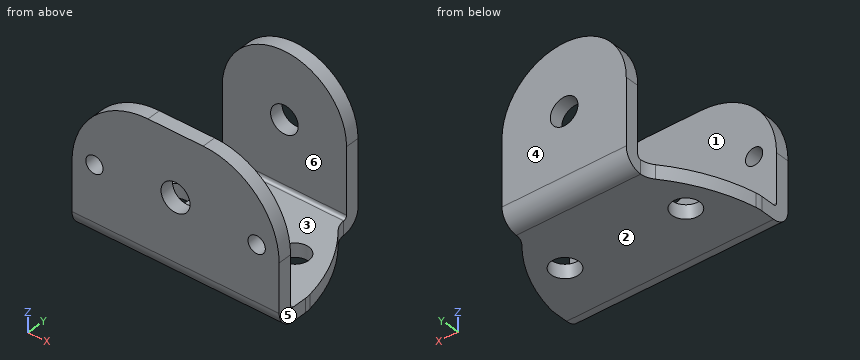
from build123d import *

# Parameters (mm, degrees)
BRIDA_BASE1_DEPTH                = 2
REDONDEO5MM_R                    = 5
REDONDEO3MM_R                    = 3
BRIDA_DE_ARISTA1_STRIP_W         = 9
BRIDA_DE_ARISTA1_STRIP_H         = 2
BRIDA_DE_ARISTA1_STRIP_CUT_DEPTH = 30
BRIDA_DE_ARISTA1_DEPTH           = 30
BRIDA_DE_ARISTA2_DEPTH           = 18
BRIDA_START                      = 2
BRIDA_DE_ARISTA2_FLAT_DEPTH      = 2
CORTAR_EXTRUIR6_REACH            = 43.255
CROQUIS26_R                      = 2
REDONDEO11MM_R                   = 11
TALADRO_ROSCADO_M32_D            = 2.5
TALADRO_ROSCADO_M32_DEPTH        = 20.65
TALADRO_ROSCADO_M32_TIP          = 0.751075774
TALADRO_ROSCADO_M52_D            = 4.2
TALADRO_ROSCADO_M52_DEPTH        = 2
CORTAR_EXTRUIR7_REACH            = 42.274
CROQUIS36_R                      = 2


# Sheet-metal steps are written as plain solids
with BuildPart() as part:
    # Croquis1 → Brida base1 (new body)
    with BuildSketch(Plane.XY):
        with BuildLine():
            Line((0, 0), (30, 0))
            Line((30, 0), (30, 3))
            ThreePointArc((30, 3), (27.901523057, 9.682731068), (24, 15.5))
            Line((24, 15.5), (24, 16.5))
            Line((24, 16.5), (6, 16.5))
            Line((6, 16.5), (6, 15.5))
            ThreePointArc((6, 15.5), (2.098476943, 9.682731068), (0, 3))
            Line((0, 3), (0, 0))
        make_face()
    extrude(amount=-BRIDA_BASE1_DEPTH)

    # Redondeo5mm
    redondeo5mm_edges = [part.edges().sort_by_distance(p)[0] for p in [
        (0, 3, -1),
        (30, 3, -1),
    ]]
    fillet(redondeo5mm_edges, radius=REDONDEO5MM_R)

    # Redondeo3mm
    # the kernel refuses this fillet: 3 mm, written as the material it adds along each edge
    with BuildSketch(Plane(origin=(24, 15.5, 0), x_dir=(0, 1, 0), z_dir=(0, 0, -1))) as redondeo3mm_piece_1:
        with BuildLine():
            CenterArc((1.118262022, 2.997668109), REDONDEO3MM_R, 230.394906527, 37.345869832)
            Line((-0.794215431, 0.686298387), (-0.83246498, 0.640070993))
            ThreePointArc((-0.83246498, 0.640070993), (-0.432666371, 0.301999114), (-0.040192089, -0.044548805))
            Line((-0.040192089, -0.044548805), (0, -0.06))
            ThreePointArc((0, -0.06), (0.5, -0.06), (0.99763476, -0.059953362))
            Line((0.99763476, -0.059953362), (1, 0))
        make_face()
    extrude(amount=2)
    with BuildSketch(Plane(origin=(6, 15.5, 0), x_dir=(-0.6538299662985165, -0.75664151034032, 0), z_dir=(0, 0, -1))) as redondeo3mm_piece_2:
        with BuildLine():
            CenterArc((1.113841774, 2.999313346), REDONDEO3MM_R, 231.428232408, 37.345869832)
            Line((-0.75664151, 0.653829966), (-0.794051176, 0.606920299))
            ThreePointArc((-0.794051176, 0.606920299), (-0.417550553, 0.281516493), (-0.039229798, -0.045398491))
            Line((-0.039229798, -0.045398491), (0.001283659, -0.059986267))
            ThreePointArc((0.001283659, -0.059986267), (0.524829407, -0.054385173), (1.048375155, -0.059986267))
            Line((1.048375155, -0.059986267), (1.049658814, 0))
        make_face()
    extrude(amount=2)

    # Brida de arista1 strip (across the edge) → Brida de arista1 strip cut (cut)
    with BuildSketch(Plane.YZ):
        with Locations((-4, -1)):
            Rectangle(BRIDA_DE_ARISTA1_STRIP_W, BRIDA_DE_ARISTA1_STRIP_H)
    extrude(amount=BRIDA_DE_ARISTA1_STRIP_CUT_DEPTH, mode=Mode.SUBTRACT)

    # Brida de arista1 section (across the edge) → Brida de arista1 (add)
    with BuildSketch(Plane.YZ):
        with BuildLine():
            Line((-2, 0.5), (-2, 18.5))
            Line((-2, 18.5), (0, 18.5))
            Line((0, 18.5), (0, 0.5))
            ThreePointArc((0, 0.5), (0.146446609, 0.146446609), (0.5, 0))
            Line((0.5, 0), (0.5, -2))
            ThreePointArc((0.5, -2), (-1.267766953, -1.267766953), (-2, 0.5))
        make_face()
    extrude(amount=BRIDA_DE_ARISTA1_DEPTH)

    # Brida de arista2 bend section (across the edge) → Brida de arista2 (add)
    with BuildSketch(Plane(origin=(24, 17, 0), x_dir=(0, -1, 0), z_dir=(-1, 0, 0))):
        with BuildLine():
            Line((-2, 0.5), (0, 0.5))
            ThreePointArc((0, 0.5), (0.146446609, 0.146446609), (0.5, 0))
            Line((0.5, 0), (0.5, -2))
            ThreePointArc((0.5, -2), (-1.267766953, -1.267766953), (-2, 0.5))
        make_face()
    extrude(amount=BRIDA_DE_ARISTA2_DEPTH)

    # Brida de arista2 profile (on flange) → Brida de arista2 flat (add)
    with BuildSketch(Plane(origin=(0, 17, 0), x_dir=(-1, 0, 0), z_dir=(0, 1, 0)).offset(BRIDA_START)):
        with BuildLine():
            ThreePointArc((-6, 10), (-15, 19), (-24, 10))
            Line((-24, 10), (-24, 0.5))
            Line((-24, 0.5), (-6, 0.5))
            Line((-6, 0.5), (-6, 10))
        make_face()
    extrude(amount=-BRIDA_DE_ARISTA2_FLAT_DEPTH)

    # Croquis26 → Cortar-Extruir6 (cut, up to next)
    with BuildSketch(Plane(origin=(0, 0, -2), x_dir=(-1, 0, 0), z_dir=(0, 0, -1)), mode=Mode.PRIVATE) as cortar_extruir6_sk1:
        with Locations((-6.25, 8.3)):
            Circle(CROQUIS26_R)
    cortar_extruir6_tool1 = extrude(cortar_extruir6_sk1.sketch, amount=-CORTAR_EXTRUIR6_REACH, mode=Mode.PRIVATE) & part.part
    # Croquis26 → Cortar-Extruir6 (cut, up to next)
    with BuildSketch(Plane(origin=(0, 0, -2), x_dir=(-1, 0, 0), z_dir=(0, 0, -1)), mode=Mode.PRIVATE) as cortar_extruir6_sk2:
        with Locations((-23.75, 8.3)):
            Circle(CROQUIS26_R)
    cortar_extruir6_tool2 = extrude(cortar_extruir6_sk2.sketch, amount=-CORTAR_EXTRUIR6_REACH, mode=Mode.PRIVATE) & part.part
    add(cortar_extruir6_tool1.solids().sort_by_distance((6.25, 8.3, -2))[0], mode=Mode.SUBTRACT)
    add(cortar_extruir6_tool2.solids().sort_by_distance((23.75, 8.3, -2))[0], mode=Mode.SUBTRACT)

    # Redondeo11mm
    redondeo11mm_edges = [part.edges().sort_by_distance(p)[0] for p in [
        (0, -1, 18.5),
        (30, -1, 18.5),
    ]]
    fillet(redondeo11mm_edges, radius=REDONDEO11MM_R)

    # Taladro roscado M32
    with Locations(Plane(origin=(0, 0, 0), x_dir=(1, 0, 0), z_dir=(0, 1, 0))):
        with Locations((3.25, -8.5), (26.75, -8.5)):
            Hole(TALADRO_ROSCADO_M32_D / 2, depth=TALADRO_ROSCADO_M32_DEPTH)
            with Locations((0, 0, -(TALADRO_ROSCADO_M32_DEPTH + TALADRO_ROSCADO_M32_TIP / 2))):  # 118° drill point
                Cone(0, TALADRO_ROSCADO_M32_D / 2, TALADRO_ROSCADO_M32_TIP, mode=Mode.SUBTRACT)

    # Taladro roscado M52
    with Locations(Plane(origin=(3.715500562, 0, 2.638137214), x_dir=(1, 0, 0), z_dir=(0, 1, 0))):
        with Locations((11.284499438, -6.861862786)):
            Hole(TALADRO_ROSCADO_M52_D / 2, depth=TALADRO_ROSCADO_M52_DEPTH)

    # Croquis36 → Cortar-Extruir7 (cut, up to next)
    with BuildSketch(Plane(origin=(0, 17, 0), x_dir=(1, 0, 0), z_dir=(0, 1, 0)), mode=Mode.PRIVATE) as cortar_extruir7_sk1:
        with Locations(Location((15, -9.5, 0), (0, 0, 270))):
            Circle(CROQUIS36_R)
    cortar_extruir7_tool1 = extrude(cortar_extruir7_sk1.sketch, amount=CORTAR_EXTRUIR7_REACH, mode=Mode.PRIVATE) & part.part
    add(cortar_extruir7_tool1.solids().sort_by_distance((15, 17, 9.5))[0], mode=Mode.SUBTRACT)


solid = part.part
Work out the finished part from the listing and answer in its coordinate system (mm). Face numbers are marked on the shaded views. A direction names the side the tool comes from. Coordinates: 2 decimals unless noted, no trailing zeros. Write each loop counter-clockwise with the first axis right and the second up, starting at its lowest first coordinate (ties: lowest second). Pieces come first, ordered by that corner, then holes. Notation, with made-up numbers: M -9.5,14 L 6.5,14 A7 cw 6.5,22 Z; hole C -12.5,-3.5 d10. An arc over 180 degrees is marked long. Answer as CSV lines item,"result". Start each with the question number.
Item 1: Section A-A on x = 15 is taken. Write down the section's boundary in (y, z), and give its area (3 significant figures).
Item 2: Consider L1, parallel to Y at x = 14.25, z = 1; L2, parallel to X at y = 18.15, z = 9.5; L3, parallel to X at y = -1, z = 8.5. Determine where each line is inside the solid, lowest interval first.
Item 3: Section C-C on y = 7 is taken. Write down the section's boundary in (x, z).
Item 4: Section B-B on x = 23 is taken. Write down the section's boundary in (y, z).
Item 5: Section D-D on z = 8.5 is taken. Write down the section's boundary in (x, y).
Item 6: Flat-ended cylindrical pins translate along their axes: P1, Ø4, axis at y = 8, z = 1, coming from the -X side; P2, Ø1, axis at x = 16.5, y = 10.5, coming from the +Z side; P3, Ø0.8, axis at y = 17.5, z = 3.5, coming from the +X side; P4, Ø2, axis at x = 3.25, z = 8.5, coming from the +Y side. Find the tip coordinate at first contact, or state that the pin passes through.
Item 7: A tool of negligible diameter and unlimited length cuts with its end or side. For the marked faces 5 and 6, from which of +Z, -Z, +X, -X, +Y, -Y can it reach the whole face along a straight path? Write none if from no direction.
Item 8: Determine the mould class of the marked faces 1, 2, 3 and 4 for opening direction Y: released by +Y, released by -Y, zero draft, split by the parting line, or undercut.
Checks:
1,outline,"M -2,0.5 A2.5 ccw 0.5,-2 L 16.5,-2 A2.5 ccw 19,0.5 L 19,7.5 L 17,7.5 L 17,0.5 A0.5 cw 16.5,0 L 0.5,0 A0.5 cw 0,0.5 L 0,7.4 L -2,7.4 Z; M -2,11.6 L 0,11.6 L 0,18.5 L -2,18.5 Z; M 17,11.5 L 19,11.5 L 19,19 L 17,19 Z"
1,area,"98.0 mm²"
2,L1,"y = -2 to 0, 17 to 19"
2,L2,"x = 6 to 13, 17 to 24"
2,L3,"x = 0.05 to 2, 4.5 to 13.15, 16.85 to 25.5, 28 to 29.95"
3,outline,"M 1,-2 L 4.73,-2 L 4.73,0 L 1,0 Z; M 7.77,-2 L 22.23,-2 L 22.23,0 L 7.77,0 Z; M 25.27,-2 L 29,-2 L 29,0 L 25.27,0 Z"
4,outline,"M -2,0.5 A2.5 ccw 0.5,-2 L 6.45,-2 L 6.45,0 L 0.5,0 A0.5 cw 0,0.5 L 0,17.75 L -2,17.75 Z; M 10.15,-2 L 16.5,-2 A2.5 ccw 19,0.5 L 19,14.12 L 17,14.12 L 17,0.5 A0.5 cw 16.5,0 L 10.15,0 Z"
5,outline,"M 0.05,-2 L 2,-2 L 2,0 L 0.05,0 Z; M 4.5,-2 L 13.15,-2 L 13.15,0 L 4.5,0 Z; M 6,17 L 13.27,17 L 13.27,19 L 6,19 Z; M 16.73,17 L 24,17 L 24,19 L 16.73,19 Z; M 16.85,-2 L 25.5,-2 L 25.5,0 L 16.85,0 Z; M 28,-2 L 29.95,-2 L 29.95,0 L 28,0 Z"
6,P1,"stops at x = 0.76"
6,P2,"stops at z = 0"
6,P3,"stops at x = 24"
6,P4,"passes through"
7,face 5,"+Z, -Z, +X, +Y, -Y"
7,face 6,"+Z, +X, -X"
8,face 1,"undercut"
8,face 2,"zero draft"
8,face 3,"undercut"
8,face 4,"released by +Y"
